```python
from build123d import *

# Parameters (mm, degrees)
SKETCH1_R           = 3.8
BOSS_EXTRUDE1_DEPTH = 2.2
SKETCH2_R           = 2
BOSS_EXTRUDE2_DEPTH = 50
CHAMFER1_SIZE       = 0.3
CUT_EXTRUDE1_DEPTH  = 2
FILLET1_R           = 1.8


with BuildPart() as part:
    # Sketch1 → Boss-Extrude1 (new body)
    with BuildSketch(Plane.XY):
        Circle(SKETCH1_R)
    extrude(amount=BOSS_EXTRUDE1_DEPTH)

    # Sketch2 → Boss-Extrude2 (add)
    with BuildSketch(Plane(origin=(0, 0, 0), x_dir=(-1, 0, 0), z_dir=(0, 0, -1))):
        Circle(SKETCH2_R)
    extrude(amount=BOSS_EXTRUDE2_DEPTH)

    # Chamfer1
    chamfer1_edges = [part.edges().sort_by_distance(p)[0] for p in [
        (2, 0, -50),
    ]]
    chamfer(chamfer1_edges, length=CHAMFER1_SIZE)

    # Sketch3 → Cut-Extrude1 (cut)
    with BuildSketch(Plane.XY.offset(2.2)):
        Polygon((0, 1.443375673), (-1.25, 0.721687836), (-1.25, -0.721687836), (0, -1.443375673), (1.25, -0.721687836), (1.25, 0.721687836), align=None)
    extrude(amount=-CUT_EXTRUDE1_DEPTH, mode=Mode.SUBTRACT)

    # Fillet1
    fillet1_edges = [part.edges().sort_by_distance(p)[0] for p in [
        (-3.8, 0, 2.2),
    ]]
    fillet(fillet1_edges, radius=FILLET1_R)


solid = part.part
```
Geometry check sheet. Reference: the model listing, model coordinates, mm. A direction names the side the tool comes from. Round coordinates to 2 decimals unless told otherwise and drop trailing zeros. Order: outer loops, then holes, each group sorted by start corner. A loop starts at its lowest first (then second) coordinate and runs counter-clockwise, first axis right, second up. Notation, with made-up numbers: M -25,53 L 9,53 A31 cw 9,81 Z; hole C 48.25,79 d8. An arc over 180 degrees is marked long. Write item = value, one per line.
Q1. Section check B-B (z = -23). Enter the section's corners in (x, y).
Answer block:
outline = C 0,0 d4
Q2. Section check A-A (y = 0). Enter the section's corners in (x, z), plus the area to 3 significant figures.
Answer block:
outline = M -3.8,0 L -2,0 L -2,-49.7 L -1.7,-50 L 1.7,-50 L 2,-49.7 L 2,0 L 3.8,0 L 3.8,0.4 A1.8 ccw 2,2.2 L 1.25,2.2 L 1.25,0.2 L -1.25,0.2 L -1.25,2.2 L -2,2.2 A1.8 ccw -3.8,0.4 Z
area = 210 mm^2
Q3. Depth check by flat-ended pin: pin 1 Ø1 at (y, z) = (1.5, -31) entering from +X; pin 2 Ø4 at (y, z) = (1.5, -39.5) entering from -X; pin 3 Ø2 at (y, z) = (0.5, -13.5) entering from +X. Enter the tip coordinate at first touch or a pass-through.
Answer block:
pin_1 = 1.73
pin_2 = -2
pin_3 = 2
Q4. Release check for a two-part mould opening along Y. For faces 1 (the cylindrical face through (0, -2, -25)), 2 (the flat face through (1.25, 0, 1)), 3 (the flat face through (0, 0, -50)) record: released by +Y, released by -Y, zero draft, split by the parting line, or undercut.
Answer block:
face_1 = split by the parting line
face_2 = undercut
face_3 = zero draft
Q5. Set-up check for faces 4 (the flat face through (-1.25, 0, 1)), 5 (the flat face through (2, -2, 0)), 6 (the cylindrical face through (-3.796, 0.167, 0.197)): record each of +Z, -Z, +X, -X, +Y, -Y from which the full face is reachable in a straight line by a thin tool's end or side.
Answer block:
face_4 = +Z
face_5 = -Z
face_6 = +Z, -Z
Q6. Scan lines: line 1 (Y direction, x = 0, z = -18); line 2 (Y direction, x = 0.75, z = -6); line 3 (Z direction, x = -2, y = 1.75). Record each from-to range of solid material in increasing order.
Answer block:
line_1 = -2 to 2
line_2 = -1.85 to 1.85
line_3 = 0 to 2.08
